Autodesk Inventor part; units mm, degrees
ref_plane "YZ Plane" through (0, 0, 0) normal (1, 0, 0) x (0, 1, 0)
ref_plane "XZ Plane" through (0, 0, 0) normal (0, 1, 0) x (-1, 0, 0)
ref_plane "XY Plane" through (0, 0, 0) normal (0, 0, 1) x (1, 0, 0)
sketch "Sketch1" plane through (0, 0, 0) normal (0, 1, 0) x (-1, 0, 0)
  circle A0 centre (0, 0) radius 51
  circle A1 centre (0, 0) radius 47.55
  circle A2 centre (0, 0) radius 54.45
  dimension "d0" = 102
  dimension "d6" = 95.1
  dimension "d7" = 108.9
extrude "Extrusion1" add sketch "Sketch1" along normal blind 30 contours A0 | A2
sketch "Sketch2" plane through (0, 30, 0) normal (0, 1, 0) x (1, 0, 0)
  line L0 (-51, 3.9837) -> (-47.55, 1.9919)
  line L1 (-47.55, 1.9919) -> (-47.55, -1.9919)
  line L2 (-47.55, -1.9919) -> (-51, -3.9837)
  line L3 (-51, -3.9837) -> (-54.45, -1.9919)
  line L4 (-54.45, -1.9919) -> (-54.45, 1.9919)
  line L5 (-54.45, 1.9919) -> (-51, 3.9837)
  circle A0 centre (0, 0) radius 54.45
  circle A1 centre (0, 0) radius 47.55
  line L6 (-51, -3.9837) -> (-47.2749, -3.9837)
  line L7 (-47.2749, -3.9837) -> (-47.2749, 3.9837)
  line L8 (-47.2749, 3.9837) -> (-51, 3.9837)
  line L9 (-51, 3.9837) -> (-51, -3.9837)
  point P0 (-51, 0)
  point P1 (-54.4128, 2.0134)
  point P2 (-54.4128, -2.0134)
  point P3 (-47.3828, -3.9837)
  point P4 (-47.55, 0)
  point P5 (-47.3828, 3.9837)
extrude "Extrusion2" cut sketch "Sketch2" against normal blind 3 contours L8 A1 L1 L0 | L9 L3 A0 L5 | L0 L1 L2 L9 | L8 L7 L6 A1 | A1 L6 L7 L8 | L2 L1 A1 L6
pattern_circular "Circular Pattern1" count 3 over 360 about axis through (0, 0, 0) along (0, 1, 0) of "Extrusion2"
sketch "Sketch3" plane through (0, 30, 0) normal (0, 1, 0) x (1, 0, 0)
  circle A0 centre (0, 0) radius 47.55
  circle A1 centre (0, 0) radius 54.45
extrude "Extrusion3" add sketch "Sketch3" along normal blind 5
sketch "Sketch4" plane through (0, 35, 0) normal (0, 1, 0) x (1, 0, 0)
  line L0 (-76.23, 0) -> (76.23, 0)
  point P0 (0, 0)
  point P1 (-51, 0)
  dimension "d22" = 51
hole "Hole1" at (-51, 35, 0) direction (0, -1, 0) diameter 4.2 depth 5
pattern_circular "Circular Pattern2" count 3 over 360 about axis through (0, 0, 0) along (0, 1, 0) of "Hole1"
sketch "Sketch5" plane through (0, 0, 0) normal (0, -1, 0) x (1, 0, 0)
  circle A0 centre (0, 0) radius 47.55
  circle A1 centre (0, 0) radius 57.192
extrude "Extrusion4" add sketch "Sketch5" along normal blind 3
chamfer "Chamfer2" distance 2.5 angle 45 1 edges at (54.45, 0, 0)
properties part number "CenterCylinder_2"
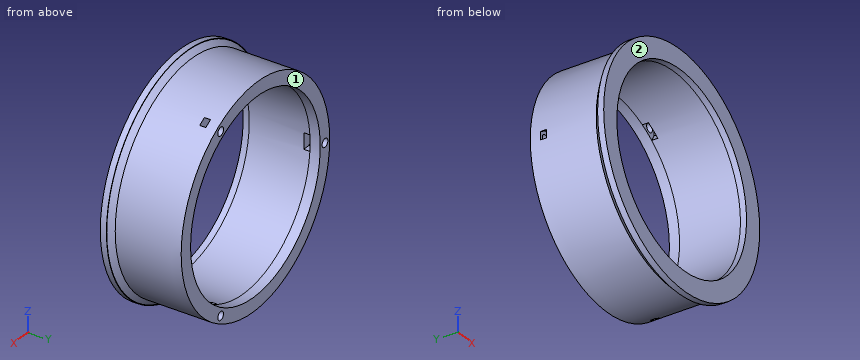
Check sheet for the modelled part. Datum: model origin and axes. Units: mm. Face numbers are marked on the shaded views. Round coordinates to 2 decimals unless told otherwise and drop trailing zeros. Loops run counter-clockwise (first coordinate to the right, second up) from the corner with the lowest first, then second, coordinate; pieces in that order, holes last. Notation, with made-up numbers: (35.5, 23) -> (47.5, 23) arc R25 ccw to (47.5, 42) -> close; hole circle Ø2 at (-33, 44.25). An arc over 180 degrees is marked (long way). Put each result on its own line as item: value. Start each with the question number.
1. Scan lines: probe 1 along X at (y, z) = (32.6, 0); probe 2 along X at (y, z) = (14, 0). Record each from-to range of solid material in increasing order.
2. Gauge pin test, flat ends, axial feed: pin 1 (4 mm diameter, centred on y = 10, z = 11, fed in from -X); pin 2 (0.9 mm diameter, centred on x = -49.5, y = 29, fed in from +Z); pin 3 (8 mm diameter, centred on x = -18, y = 12, fed in from +Z). Record the tip position at first contact, or that the pin passes through.
3. Section check B-B (y = 6). Enter the section's corners in (x, z), plus the area to 3 significant figures.
4. Draft check along Y on the marked faces 1 and 2. Enter one of: +Y half, -Y half, draft (parallel to the pull), parting line (faces both ways), or undercut.
Findings:
1. probe 1: x = -54.45 to -53.1, -48.9 to -47.55, 47.55 to 54.45
1. probe 2: x = -54.45 to -47.55, 47.55 to 54.45
2. pin 1: stops at x = -53.7
2. pin 2: stops at z = 23.64
2. pin 3: stops at z = 52.62
3. outline: circle Ø108.9 at (0, 0); hole circle Ø95.1 at (0, 0)
3. area: 2,210 mm^2
4. face 1: +Y half
4. face 2: -Y half
